from build123d import *

# Parameters (mm, degrees)
F0_W     = 20
F0_H     = 25
F1_DEPTH = 10
F3_D     = 3
F3_DEPTH = 10
F3_TIP   = 0.9012909285
F4_R     = 0.99999


# Not quite as in the source:
# - a fillet or chamfer is up to 0.001 mm smaller than in the source, because OpenCascade refuses the exact size


with BuildPart() as f1:
    # F0 (on Top) → F1 (new body)
    with BuildSketch(Plane.XY):
        with Locations((-11.3712290768, -0.8075441738)):
            Rectangle(F0_W, F0_H)
    extrude(amount=F1_DEPTH)

    # F3
    with Locations(Plane.XY.offset(10)):
        with Locations((-11.3712290768, 8.1924558262), (-11.3712290768, -9.8075441738)):
            Hole(F3_D / 2, depth=F3_DEPTH)
            with Locations((0, 0, -(F3_DEPTH + F3_TIP / 2))):  # 118° drill point
                Cone(0, F3_D / 2, F3_TIP, mode=Mode.SUBTRACT)

    # F4 (radius 1 in the source; OpenCascade refuses exactly that, so slightly less here)
    f4_edges = [f1.edges().sort_by_distance(p)[0] for p in [
        (-11.371229, -13.307544, 0),
        (-21.371229, -0.807544, 0),
        (-1.371229, -0.807544, 0),
        (-11.371229, 11.692456, 0),
        (-12.871229, -9.807544, 0),
        (-12.871229, 8.192456, 0),
    ]]
    fillet(f4_edges, radius=F4_R)


solid = f1.part
Geometry: final body of the model. Coordinates: model frame, mm. Coordinates: 2 decimals unless noted, no trailing zeros. Order: outer loops, then holes, each group sorted by start corner. A loop starts at its lowest first (then second) coordinate and runs counter-clockwise, first axis right, second up.
1) Section A-A (z = 6). Return loops of the section in (x, y).
Result sheet:
outline: (-21.37, -13.31) - (-1.37, -13.31) - (-1.37, 11.69) - (-21.37, 11.69) - close; hole circle Ø3 at (-11.37, -9.81); hole circle Ø3 at (-11.37, 8.19)
2) Ray query, probe 1 along Y at (x, z) = (-10, 3.25); probe 2 along X at (y, z) = (-10.5, 0.75); probe 3 along Y at (x, z) = (-12.25, 1). Return the intervals inside material, ascending.
Result sheet:
probe 1: y = -13.31 to -10.42, -9.2 to 7.58, 8.8 to 11.69
probe 2: x = -21.34 to -12.74, -10 to -1.4
probe 3: y = -13.31 to -11.02, -8.59 to 6.98, 9.41 to 11.69
3) Section B-B (x = -12.25). Give the number of separate pieces and of enclosed holes in the cut face, then the cut area to 3 significant figures.
Result sheet:
separate pieces: 3
enclosed holes: 0
area: 200 mm2
4) First-contact query: P1, Ø2.5, axis at x = -11.37, y = 8.19, coming from the +Z side. Flat tip, straight axial feed; report the tip coordinate or a pass-through.
Result sheet:
P1: passes through
5) Section C-C (z = 0.5). Return loops of the section in (x, y).
Result sheet:
outline: (-21.24, -13.17) - (-1.51, -13.17) - (-1.51, 11.56) - (-21.24, 11.56) - close; hole circle Ø3.27 at (-11.37, -9.81); hole circle Ø3.27 at (-11.37, 8.19)
6) Draft query along X for faces 1 (the cylindrical face through (-10.18, -10.72, 5.44)), 2 (the cylindrical face through (-21.086, -0.633, 0.301)), 3 (the flat face through (-11, -1, 0)), 4 (the cylindrical face through (-1.656, -0.633, 0.301)). Return one class per face: released by +X, released by -X, zero draft, split by the parting line, or undercut.
Result sheet:
face 1: undercut
face 2: released by -X
face 3: zero draft
face 4: released by +X
